Input: part model. Units: mm. Frame: model coordinates. A direction names the side the tool comes from. Coordinates: 2 decimals unless noted, no trailing zeros. Loops run counter-clockwise (first coordinate to the right, second up) from the corner with the lowest first, then second, coordinate; pieces in that order, holes last. Notation, with made-up numbers: (53.5, -16.75) - (96.5, -16.75) arc R25 cw to (96.5, 14.25) - close; hole circle Ø6 at (25, 27.5). An arc over 180 degrees is marked (long way). Use one line per item in the form item = value.
from build123d import *

# Parameters (mm, degrees)
F0_W     = 85.5915052816
F0_H     = 9.4415829517
F1_DEPTH = 150
F2_DEPTH = 150
F4_R     = 5.981115506
F5_DEPTH = 7.62


# Not quite as in the source:
# - a feature of the source that left no trace in its solid (it failed there, or was rolled back) is left out


with BuildPart() as f1:
    # F0 (on Right) → F1 (new body)
    with BuildSketch(Plane.YZ):
        with Locations((-29.4651468284, 4.7207914758)):
            Rectangle(F0_W, F0_H)
    extrude(amount=F1_DEPTH)

    # F2 (cut): a face of the model
    f2_faces = [f1.faces().sort_by_distance(p)[0] for p in [
        (75, -72.2608994693, 4.7207914758),
    ]]
    extrude(f2_faces, amount=F2_DEPTH, mode=Mode.SUBTRACT)

    # F4 (on face) → F5 (join)
    with BuildSketch(Plane.XY.offset(9.4415829517)):
        with Locations((59.6557557583, -27.7189966291)):
            Circle(F4_R)
    extrude(amount=F5_DEPTH)


solid = f1.part
Q1. Set-up query: faces 1 (the flat face through (60, -28, 17.062)), 2 (the cylindrical face through (53.68, -27.46, 13.2)). Return all of +Z, -Z, +X, -X, +Y, -Y with unobstructed straight access to the full face (end or side cutting, diameter ignored); none if empty.
Check values:
face_1 = +Z, +X, -X, +Y, -Y
face_2 = +Z
Q2. Cut plane C-C, the plane z = 11.75. Return loops of the section in (x, y).
Check values:
outline = circle Ø11.96 at (59.66, -27.72)
Q3. First-contact query: P1, Ø5, axis at x = 88.5, y = 3, coming from the +Z side. Flat tip, straight axial feed; report the tip coordinate or a pass-through.
Check values:
P1 = 9.44
Q4. Cut plane B-B, the plane x = 22.5. Return loops of the section in (y, z), then the cut area to 3 significant figures.
Check values:
outline = (-72.26, 0) - (13.33, 0) - (13.33, 9.44) - (-72.26, 9.44) - close
area = 808 mm²
Q5. Cut plane A-A, the plane y = -5. Return loops of the section in (x, z), then the cut area to 3 significant figures.
Check values:
outline = (0, 0) - (150, 0) - (150, 9.44) - (0, 9.44) - close
area = 1,420 mm²
Q6. Ray query, line 1 along Z through (x, y) = (143, -36.5); line 2 along Y through (x, z) = (58.5, 13.75). Return the intervals inside material, ascending. Write a range as [from, to].
Check values:
line_1 = [0, 9.44]
line_2 = [-33.59, -21.85]
